Input: part model. Units: mm. Frame: model coordinates. Give positions to 0.01 mm unless a question says otherwise; leave off trailing zeros. Order: outer loops, then holes, each group sorted by start corner. A loop starts at its lowest first (then second) coordinate and runs counter-clockwise, first axis right, second up. Notation, with made-up numbers: (15, -8) - (41, -8) arc R23 ccw to (41, 23) - close; hole circle Ø5 at (38.5, -18). An arc over 180 degrees is marked (long way). Use a Markdown table: item, result.
from build123d import *

# Parameters (mm, degrees)
BASE_EXTRUDE_DEPTH = 0.8
FILLET1_R          = 0.9
SKETCH2_R          = 0.6
CUT_EXTRUDE1_DEPTH = 9.260801437


with BuildPart() as part:
    # Sketch1 → Base-Extrude (new body)
    with BuildSketch(Plane.XY):
        with BuildLine():
            Line((-0.6, -3.752332608), (-0.6, -6.552332608))
            Line((-0.6, -6.552332608), (-3, -6.129147854))
            Line((-3, -6.129147854), (-3, -3.724921052))
            ThreePointArc((-3, -3.724921052), (0, 5.2), (3, -3.724921052))
            Line((3, -3.724921052), (3, -6.129147854))
            Line((3, -6.129147854), (0.6, -6.552332608))
            Line((0.6, -6.552332608), (0.6, -3.752332608))
            ThreePointArc((0.6, -3.752332608), (0, 3.8), (-0.6, -3.752332608))
        make_face()
    extrude(amount=BASE_EXTRUDE_DEPTH)

    # Fillet1
    fillet1_edges = [part.edges().sort_by_distance(p)[0] for p in [
        (3, -6.129147854, 0.4),
        (-3, -6.129147854, 0.4),
    ]]
    fillet(fillet1_edges, radius=FILLET1_R)

    # Sketch2 → Cut-Extrude1 (cut, through all)
    with BuildSketch(Plane.XY.offset(0.8)):
        with Locations((2.1, -5.373958186)):
            Circle(SKETCH2_R)
    cut_extrude1 = extrude(amount=-CUT_EXTRUDE1_DEPTH, mode=Mode.SUBTRACT)

    # Mirror1: Cut-Extrude1 across plane
    add(cut_extrude1.mirror(Plane(origin=(0, 0, 0), x_dir=(0, 0, 1), z_dir=(1, 0, 0))), mode=Mode.SUBTRACT)


solid = part.part
1. Section query D-D (y = -1). Return loops of the section in (x, z).
Response:
| item | result |
|---|---|
| outline | (-4.81, 0) - (-3.67, 0) - (-3.67, 0.8) - (-4.81, 0.8) - close; (3.67, 0) - (4.81, 0) - (4.81, 0.8) - (3.67, 0.8) - close |
2. Section query C-C (x = -2). Return loops of the section in (y, z).
Response:
| item | result |
|---|---|
| outline | (-6.31, 0) - (-5.97, 0) - (-5.97, 0.8) - (-6.31, 0.8) - close; (-4.78, 0) - (-3.23, 0) - (-3.23, 0.8) - (-4.78, 0.8) - close; (3.23, 0) - (4.78, 0) - (4.78, 0.8) - (3.23, 0.8) - close |
3. Mould query, pull axis Y, two halves, no side actions, for faces 1 (the face through (1.97, -5.96, 0.41)), 2 (the face through (2.3, 3.3, 0)), 3 (the face through (-0.173, 5.197, 0.394)), 4 (the face through (-1.97, -5.96, 0.41)). Classes: pulls with the +Y half, pulls with the -Y half, needs draft (parallel to the pull), parting line crosses it, or undercut.
Response:
| item | result |
|---|---|
| face 1 | undercut |
| face 2 | needs draft |
| face 3 | parting line crosses it |
| face 4 | undercut |
4. Section query A-A (y = -4.25). Return loops of the section in (x, z), then the cut area to 3 significant figures.
Response:
| item | result |
|---|---|
| outline | (-3, 0) - (-0.6, 0) - (-0.6, 0.8) - (-3, 0.8) - close; (0.6, 0) - (3, 0) - (3, 0.8) - (0.6, 0.8) - close |
| area | 3.84 mm^2 |
5. Material intervals for line 1 along X through (y, z) = (-5, 0.15); line 2 along Y through (x, z) = (-2.1, 0.2); line 3 along Y through (x, z) = (-2.25, 0.1), sorted ascending.
Response:
| item | result |
|---|---|
| line 1 | x = -3 to -2.57, -1.63 to -0.6, 0.6 to 1.63, 2.57 to 3 |
| line 2 | y = -6.29 to -5.97, -4.77 to -3.17, 3.17 to 4.73 |
| line 3 | y = -6.26 to -5.95, -4.79 to -3.06, 3.06 to 4.66 |
6. Pin query (flat end, axial travel): pin 1 (4.5 mm diameter, centred on x = 0, y = 0, fed in from +Z). Return the tip coordinate at first contact, or that it passes through.
Response:
| item | result |
|---|---|
| pin 1 | passes through |
7. Section query B-B (z = 0.6). Return loops of the section in (x, y).
Response:
| item | result |
|---|---|
| outline | (-3, -5.37) arc R0.9 ccw to (-2.26, -6.26) - (-0.6, -6.55) - (-0.6, -3.75) arc R3.8 cw (long way) to (0.6, -3.75) - (0.6, -6.55) - (2.26, -6.26) arc R0.9 ccw to (3, -5.37) - (3, -3.72) arc R4.97 ccw (long way) to (-3, -3.72) - close; hole circle Ø1.2 at (-2.1, -5.37); hole circle Ø1.2 at (2.1, -5.37) |
